Input: part model. Units: mm. Frame: model coordinates. A direction names the side the tool comes from. Give positions to 0.01 mm unless a question says otherwise; leave off trailing zeros. Loops run counter-clockwise (first coordinate to the right, second up) from the corner with the lowest first, then second, coordinate; pieces in that order, holes last. Notation, with made-up numbers: (37.5, 86.5) - (63.5, 86.5) arc R19 ccw to (63.5, 96.5) - close; hole circle Ø1 at (-10, 57.25). An arc over 180 degrees is marked (long way). Answer as a JSON object with one key per item and string values.
Autodesk Inventor part; units mm, degrees
ref_plane "Work Plane1" through (-4.0767, -4.0767, 5.08) normal (0, 0, -1) x (0, 1, 0)
ref_plane "YZ Plane" through (0, 0, 0) normal (1, 0, 0) x (0, 1, 0)
ref_plane "XZ Plane" through (0, 0, 0) normal (0, 1, 0) x (-1, 0, 0)
sketch "Sketch1" plane through (0, 0, 0) normal (0, 0, 1) x (1, 0, 0)
  arc A0 (-7.62, 0) -> (7.62, 0) centre (0, 0) ccw
  line L0 (1.0603, 17.7117) -> (-0.8757, 17.7117) construction
  line L1 (-7.62, 0) -> (7.62, 0)
  line L2 (7.62, 0) -> (7.62, 14.9733)
  line L3 (7.62, 14.9733) -> (-7.62, 14.9733)
  line L4 (-7.62, 14.9733) -> (-7.62, 0)
  dimension "d0" = 15.24
  dimension "d6" = 14.9733
ref_plane "Work Plane1" through (-4.0767, -4.0767, 5.08) normal (0, 0, -1) x (0, 1, 0)
extrude "Extrusion1" add sketch "Sketch1" along normal up to surface (5.08 mm away)
sketch "Sketch2" plane through (7.62, 0, 0) normal (1, 0, 0) x (0, 0, -1)
  circle A0 centre (-4.1045, 11.2117) radius 2 construction
  arc A1 (-0.3326, 11.2117) -> (-7.4701, 9.5087) centre (-4.1045, 11.2117) ccw
  circle A2 centre (-4.1045, 11.2117) radius 6.5 construction
  line L0 (-5.08, 0) -> (-5.08, 14.9733)
  line L1 (-5.08, 4.7853) -> (-7.4701, 9.5087)
  line L2 (-5.08, 4.7853) -> (-0.3326, 4.7853)
  line L3 (-0.3326, 4.7853) -> (-0.3326, 11.2117)
  point P0 (0, 0)
  dimension "d3" = 7.5438
extrude "Extrusion2" add sketch "Sketch2" against normal up to surface (15.24 mm away)
sketch "Sketch3" plane through (0, 0, 5.08) normal (0, 0, 1) x (1, 0, 0)
  circle A0 centre (0, 0) radius 4.0767 construction
  line L0 (3.0923, 15.6797) -> (3.0923, 6.7437) construction
  line L1 (-2.9077, 6.7437) -> (-2.9077, 15.6797) construction
  line L2 (3.7273, 15.6797) -> (3.7273, 6.7437) construction
  line L3 (-3.5427, 6.7437) -> (-3.5427, 15.6797) construction
  line L4 (7.62, 14.9733) -> (-7.62, 14.9733)
  line L5 (0, 4.0767) -> (3.7273, 4.0767)
  line L6 (3.7273, 4.0767) -> (3.7273, 14.9733)
  line L7 (0, 4.0767) -> (-3.5427, 4.0767)
  line L8 (-3.5427, 4.0767) -> (-3.5427, 14.9733)
  line L9 (3.7273, 15.2774) -> (-3.5427, 15.2774)
  line L10 (-3.5427, 14.9733) -> (-3.5427, 15.2774)
  line L11 (3.7273, 14.9733) -> (3.7273, 15.2774)
  dimension "d7" = 0.635
  dimension "d8" = 0.635
extrude "Extrusion3" cut sketch "Sketch3" along normal through all both and the other way through all
sketch "Sketch4" plane through (7.62, 0, 0) normal (1, 0, 0) x (0, 0, -1)
  arc A0 (-5.08, 14.8553) -> (-7.4701, 9.5087) centre (-4.1045, 11.2117) ccw construction
  circle A1 centre (-4.1045, 11.2117) radius 2.1844
  point P0 (0, 0)
  point P1 (-5.08, 7.5681)
  dimension "d11" = 4.3688
extrude "Extrusion4" cut sketch "Sketch4" against normal through all
sketch "Sketch5" plane through (0, 0, 5.08) normal (0, 0, 1) x (1, 0, 0)
  circle A0 centre (0, 0) radius 1.9685
  dimension "d14" = 3.937
extrude "Extrusion5" cut sketch "Sketch5" against normal through all
equation "\"d12\" = d11"
properties part number "omni wheel short low channel mount"
Item 1: Material intervals for line 1 (Y direction, x = 0, z = 3); line 2 (X direction, y = 7.75, z = 5.75); line 3 (Z direction, x = 2, y = -2.25), sorted ascending. Write a range as [from, to].
Geometry check:
{"line 1": "y = [-7.62, -1.97], [1.97, 4.08]", "line 2": "x = [-7.62, -3.54], [3.73, 7.62]", "line 3": "z = [0, 5.08]"}
Item 2: Cut plane C-C (x = 6). Return loops of the section in (y, z), then the cut area to 3 significant figures.
Geometry check:
{"outline": "(-4.7, 0) - (14.97, 0) - (14.97, 3.83) arc R3.77 ccw to (14.97, 4.38) - (14.97, 5.08) - (14.86, 5.08) arc R3.77 ccw to (9.51, 7.47) - (4.79, 5.08) - (-4.7, 5.08) - close; hole circle Ø4.37 at (11.21, 4.1)", "area": "103 mm2"}
Item 3: Cut plane D-D (z = 5.75). Return loops of the section in (x, y), then the cut area to 3 significant figures.
Geometry check:
{"outline": "(-7.62, 6.11) - (-3.54, 6.11) - (-3.54, 9.78) - (-7.62, 9.78) - close; (-7.62, 12.65) - (-3.54, 12.65) - (-3.54, 14.61) - (-7.62, 14.61) - close; (3.73, 6.11) - (7.62, 6.11) - (7.62, 9.78) - (3.73, 9.78) - close; (3.73, 12.65) - (7.62, 12.65) - (7.62, 14.61) - (3.73, 14.61) - close", "area": "44.8 mm2"}
Item 4: Mould query, pull axis Y, two halves, no side actions, for faces 1 (the face through (5.701, 7.114, 6.258)), 2 (the face through (0, -3, 5.08)), 3 (the face through (5.701, 11.308, 6.287)), 4 (the face through (-0.43, -1.92, 2.58)). Classes: released by +Y, released by -Y, zero draft, split by the parting line, or undercut.
Geometry check:
{"face 1": "released by -Y", "face 2": "zero draft", "face 3": "undercut", "face 4": "undercut"}
Item 5: Cut plane A-A (x = 0). Return loops of the section in (y, z), then the cut area to 3 significant figures.
Geometry check:
{"outline": "(-7.62, 0) - (-1.97, 0) - (-1.97, 5.08) - (-7.62, 5.08) - close; (1.97, 0) - (4.08, 0) - (4.08, 5.08) - (1.97, 5.08) - close", "area": "39.4 mm2"}
Item 6: Access query for faces 5 (the face through (0.17, -7.62, 2.5)), 6 (the face through (-3.543, 8, 3)). Directions: +Z, -Z, +X, -X, +Y, -Y. A direction counts if a zero-diameter tool reaches every point of the face in a straight line with its end or side. Return the directions, or none.
Geometry check:
{"face 5": "+Z, -Z, -Y", "face 6": "+Z, -Z, +Y"}
Item 7: Contact query for flat-ended pins moving along their axis: P1, Ø1.9, axis at x = -6.5, z = 2.5, coming from the +Y side; P2, Ø2.5, axis at x = -1, z = 2, coming from the +Y side; P3, Ø6.5, axis at x = 0, y = 0, coming from the +Z side; P4, Ø2.5, axis at y = 11.5, z = 3, coming from the +X side. Output: stop coordinate, or through.
Geometry check:
{"P1": "stops at y = 14.97", "P2": "stops at y = 4.08", "P3": "stops at z = 5.08", "P4": "stops at x = 7.62"}
Item 8: Cut plane B-B (z = 2.5). Return loops of the section in (x, y), then the cut area to 3 significant figures.
Geometry check:
{"outline": "(-7.62, 0) arc R7.62 ccw to (7.62, 0) - (7.62, 9.73) - (3.73, 9.73) - (3.73, 4.08) - (-3.54, 4.08) - (-3.54, 9.73) - (-7.62, 9.73) - close; (-7.62, 12.69) - (-3.54, 12.69) - (-3.54, 14.97) - (-7.62, 14.97) - close; (3.73, 12.69) - (7.62, 12.69) - (7.62, 14.97) - (3.73, 14.97) - close; hole circle Ø3.94 at (0, 0)", "area": "204 mm2"}
